For this review, take the finished solid that the model builds, in its own axes (mm). Face numbers are marked on the shaded views. A direction names the side the tool comes from. Give positions to 0.01 mm unless a question says otherwise; leave off trailing zeros. Write each loop counter-clockwise with the first axis right and the second up, starting at its lowest first coordinate (ties: lowest second). Pieces come first, ordered by that corner, then holes. Notation, with made-up numbers: (1.5, 48.5) -> (15.5, 48.5) arc R34 ccw to (15.5, 87.5) -> close; hole circle Ø5 at (54.5, -19). An arc over 180 degrees is marked (long way). Write item = value, one per line.
```python
from build123d import *

# Parameters (mm, degrees)
PAD_DEPTH    = 60
CHAMFER_SIZE = 2
FILLET_R     = 2


with BuildPart() as part:
    # Sketch → Pad (new body)
    with BuildSketch(Plane.YZ):
        Polygon((20, 18.5), (20, -18.5), (0, -18.5), (0, -38.5), (-20, -18.5), (-20, 18.5), align=None)
    extrude(amount=PAD_DEPTH)

    # Chamfer
    chamfer_edges = [part.edges().sort_by_distance(p)[0] for p in [
        (0, 20, 0),
        (0, 10, -18.5),
        (0, 0, -28.5),
        (0, -10, -28.5),
        (0, -20, 0),
        (0, 0, 18.5),
        (60, 20, 0),
        (60, 10, -18.5),
        (60, 0, -28.5),
        (60, -10, -28.5),
        (60, -20, 0),
        (60, 0, 18.5),
    ]]
    chamfer(chamfer_edges, length=CHAMFER_SIZE)

    # Fillet
    fillet_edges = [part.edges().sort_by_distance(p)[0] for p in [
        (30, 0, -38.5),
        (30, 20, -18.5),
        (30, 20, 18.5),
        (30, -20, 18.5),
        (30, -20, -18.5),
    ]]
    fillet(fillet_edges, radius=FILLET_R)


solid = part.part
```
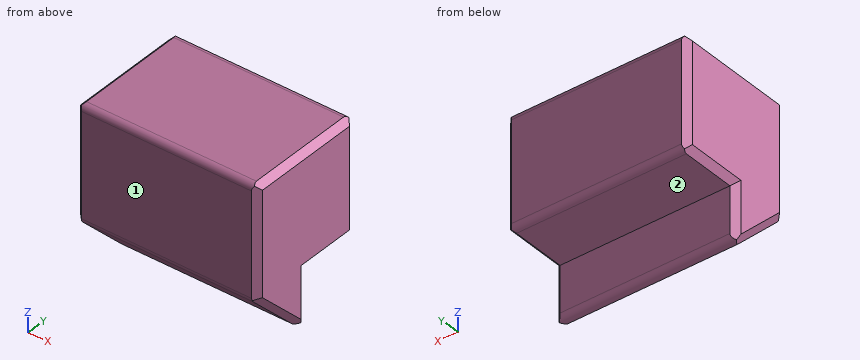
(1) To check wall thickness, follow probe 1 along Z at (x, y) = (38, 15); probe 2 along Z at (x, y) = (50, -7); probe 3 along Y at (x, z) = (37.5, -26). State the ranges of each line that lie inside material, in increasing order.
Answers below:
probe_1 = -18.5 to 18.5
probe_2 = -31.5 to 18.5
probe_3 = -12.5 to 0
(2) Tool access review of the marked faces 1 and 2: name each direction out of +Z, -Z, +X, -X, +Y, -Y from which nothing blocks a thin tool from reaching the whole face with its end or side.
Answers below:
face_1 = +Z, -Z, +X, -X, -Y
face_2 = -Z, +X, -X, +Y
(3) Take a section at A-A (y = 16). Write out the cut boundary in (x, z).
Answers below:
outline = (0, -16.5) -> (2, -18.5) -> (58, -18.5) -> (60, -16.5) -> (60, 16.5) -> (58, 18.5) -> (2, 18.5) -> (0, 16.5) -> close
(4) Take a section at B-B (x = 27). Write out the cut boundary in (y, z), plus the area to 3 significant figures.
Answers below:
outline = (-20, -17.67) arc R2 ccw to (-19.41, -19.09) -> (-3.41, -35.09) arc R2 ccw to (0, -33.67) -> (0, -18.5) -> (18, -18.5) arc R2 ccw to (20, -16.5) -> (20, 16.5) arc R2 ccw to (18, 18.5) -> (-18, 18.5) arc R2 ccw to (-20, 16.5) -> close
area = 1,670 mm^2
(5) For pin 1 (1 mm diameter, centred on x = 24.5, y = 13.5, fed in from -Z); pin 2 (12 mm diameter, centred on x = 36.5, z = -27.5, fed in from -Y); pin 3 (6 mm diameter, centred on x = 30, y = -11.5, fed in from -Z), all flat-tipped, find the tip position at first contact; note any pin that passes through.
Answers below:
pin_1 = -18.5
pin_2 = -17
pin_3 = -30
(6) Take a section at C-C (z = -24.5). Write out the cut boundary in (x, y).
Answers below:
outline = (0, -11.17) -> (2, -14) -> (58, -14) -> (60, -11.17) -> (60, -2) -> (58, 0) -> (2, 0) -> (0, -2) -> close
